The model under review builds one solid part; all positions refer to its coordinate system, in mm. A direction names the side the tool comes from. Give positions to 0.01 mm unless a question says otherwise; leave off trailing zeros. Loops run counter-clockwise (first coordinate to the right, second up) from the corner with the lowest first, then second, coordinate; pieces in that order, holes last. Notation, with made-up numbers: M 59.5,44.5 L 105.5,44.5 A31 ccw 105.5,72.5 Z; hole C 51,5 d2. An arc over 180 degrees is marked long. One line per item, written item: value. Start each with the question number.
Q1. To check wall thickness, follow line 1 along Y through (x, z) = (0, 5); line 2 along Z through (x, y) = (4.5, -14); line 3 along Y through (x, z) = (4.5, 2). State the ranges of each line that lie inside material, in increasing order. Write a range as from..to.
Q2. For pin 1 (1.6 mm diameter, centred on y = -1.21, z = 2.5, fed in from +X), flat-tipped, find the tip position at first contact; note if it passes through.
Q3. We need section A-A on x = 4.5. Write out the cut boundary in (y, z), plus the area to 3 significant figures.
Q4. We need section B-B on z = 7.5. Give the number of separate pieces and of enclosed holes in the cut face, plus the area to 3 significant figures.
Q5. Mouldability with a two-part tool opening along X and no side actions: class faces 1 (the face through (13.5, -3, 4)), 2 (the face through (-1, 0.32, 4.44)), 3 (the face through (4, 0, 0)) as released by +X, released by -X, zero draft, split by the parting line, or undercut.
Q6. For faces 4 (the face through (11, -1, 3)), 5 (the face through (13.199, 2.215, 4.437)), 6 (the face through (4.61, -13.21, 2.72)), list the 3-axis set-ups (+Z, -Z, +X, -X, +Y, -Y) from which the entire face can be reached by the end or side of a thin tool; tool diameter is ignored.
Autodesk Inventor part; units mm, degrees
ref_plane "Work Plane1" through (0, -22.25, 0) normal (0, 1, 0) x (1, 0, 0)
ref_plane "YZ Plane" through (0, 0, 0) normal (1, 0, 0) x (0, 1, 0)
ref_plane "XZ Plane" through (0, 0, 0) normal (0, 1, 0) x (-1, 0, 0)
sketch "Sketch1" plane through (0, 0, 0) normal (0, 0, 1) x (1, 0, 0)
  circle A0 centre (9, 0) radius 1
  circle A1 centre (0, 0) radius 1
  line L0 (0, 2.5) -> (9, 2.5)
  arc A2 (0, 2.5) -> (-2.5, 0) centre (0, 0) ccw
  arc A3 (11.5, 0) -> (9, 2.5) centre (9, 0) ccw
  arc A4 (-3.2143, -2.5754) -> (-2.5, 0) centre (-7.5, 0) ccw
  arc A5 (11.5, 0) -> (12.2143, -2.5754) centre (16.5, 0) ccw
  arc A6 (-3.2143, -2.5754) -> (-4.1458, -4.7111) centre (4.5, -7.2111) ccw
  line L1 (-8.5, -4.7111) -> (-4.1458, -4.7111)
  line L2 (13.1458, -4.7111) -> (17.5, -4.7111)
  line L3 (17.5, -9.7111) -> (13.1458, -9.7111)
  line L4 (-4.1458, -9.7111) -> (-8.5, -9.7111)
  line L5 (17.5, -7.9611) -> (10.4529, -7.9611)
  line L6 (-1.4529, -7.9611) -> (-8.5, -7.9611)
  line L7 (-8.5, -6.4611) -> (-1.4529, -6.4611)
  line L8 (10.4529, -6.4611) -> (17.5, -6.4611)
  arc A7 (-4.1458, -9.7111) -> (13.1458, -9.7111) centre (4.5, -7.2111) ccw
  arc A8 (13.1458, -4.7111) -> (12.2143, -2.5754) centre (4.5, -7.2111) ccw
  arc A9 (-1.4529, -7.9611) -> (10.4529, -7.9611) centre (4.5, -7.2111) ccw
  arc A10 (10.4529, -6.4611) -> (-1.4529, -6.4611) centre (4.5, -7.2111) ccw
  line L9 (17.5, -4.7111) -> (17.5, -6.4611)
  line L10 (17.5, -7.9611) -> (17.5, -9.7111)
  line L11 (-8.5, -9.7111) -> (-8.5, -7.9611)
  line L12 (-8.5, -6.4611) -> (-8.5, -4.7111)
extrude "Extrusion1" add sketch "Sketch1" along normal blind 5
sketch "Sketch2" plane through (13.1458, -9.7111, 0) normal (0, -1, 0) x (1, 0, 0)
  line L0 (4.3542, 0) -> (4.3542, 5)
  line L1 (0, 0) -> (0, 5)
  circle A0 centre (2.1771, 2.5) radius 0.9
  circle A1 centre (-19.4687, 2.5) radius 0.9
  point P0 (-13.1458, 0)
  dimension "d13" = 1.8
extrude "Extrusion2" cut sketch "Sketch2" against normal blind 5
fillet "Fillet1" radius 0.8 8 edges at (17.5, -4.7111, 2.5) (17.5, -9.7111, 2.5) (-8.5, -4.7111, 2.5) (-8.5, -9.7111, 2.5) (17.5, -6.4611, 2.5) (17.5, -7.9611, 2.5) (-8.5, -7.9611, 2.5) (-8.5, -6.4611, 2.5)
fillet "Fillet2" radius 0.8 4 edges at (-1.4529, -6.4611, 2.5) (10.4529, -6.4611, 2.5) (10.4529, -7.9611, 2.5) (-1.4529, -7.9611, 2.5)
sketch "Sketch3" plane through (0, 0, 5) normal (0, 0, 1) x (1, 0, 0)
  arc A0 (11.5, 0) -> (9, 2.5) centre (9, 0) ccw
  line L0 (14.4229, -6.4611) -> (14.4229, -4.7111)
  line L1 (9, 2.5) -> (14.4229, 2.5)
  line L2 (14.4229, 2.5) -> (14.4229, -4.7111)
  line L3 (14.4229, -4.7111) -> (9, -4.7111)
  line L4 (9, -4.7111) -> (9, 2.5)
  arc A1 (13.1458, -4.7111) -> (12.2143, -2.5754) centre (4.5, -7.2111) ccw
  arc A2 (11.5, 0) -> (12.2143, -2.5754) centre (16.5, 0) ccw
  point P0 (0, 0)
extrude "Extrusion3" add sketch "Sketch3" against normal blind 5 contours A0 L1 L2 L3 A1 A2
sketch "Sketch4" plane through (14.4229, -4.7111, 5) normal (1, 0, 0) x (0, 0, -1)
  line L0 (0, 0) -> (0, 7.2111)
  line L1 (2.5, 0) -> (0, 0)
  line L2 (5, 0) -> (2.5, 0)
  line L3 (5, 7.2111) -> (5, 0)
  line L4 (0, 7.2111) -> (5, 7.2111)
  point P0 (5, 4.7111)
extrude "Extrusion4" cut sketch "Sketch4" against normal blind 0.923
sketch "Sketch5" plane through (13.4999, -4.7111, 5) normal (1, 0, 0) x (0, 0, -1)
  line L0 (0, 3.5) -> (5, 3.5)
  circle A0 centre (2.5, 3.5) radius 0.9
  point P0 (5, 4.7111)
  dimension "d25" = 1.8
extrude "Extrusion5" cut sketch "Sketch5" against normal blind 2.5
fillet "Fillet3" radius 1 1 edges at (13.4999, 2.5, 2.5)
sketch "Sketch6" plane through (0, 0, 5) normal (0, 0, 1) x (1, 0, 0)
  arc A0 (-1.342, -8.5787) -> (10.342, -8.5787) centre (4.5, -7.2111) ccw
  circle A1 centre (4.5, -7.2111) radius 6
  circle A2 centre (4.5, -7.2111) radius 9
  line L0 (13.4999, -4.7111) -> (13.4999, 1.5)
  line L1 (13.4999, -4.7111) -> (17.88, -4.7111)
  line L2 (17.88, -4.7111) -> (17.88, -10.4948)
  line L3 (17.88, -10.4948) -> (13.4999, -10.4948)
  line L4 (13.4999, -10.4948) -> (13.4999, -4.7111)
  line L5 (-4.1458, -4.7111) -> (-7.7, -4.7111)
  line L6 (-4.1458, -4.7111) -> (-9.7441, -4.7111)
  line L7 (-9.7441, -4.7111) -> (-9.7441, -9.7121)
  line L8 (-9.7441, -9.7121) -> (-4.1458, -9.7121)
  line L9 (-4.1458, -9.7121) -> (-4.1458, -4.7111)
  line L10 (13.4999, -10.4948) -> (12.8796, -10.4948)
  point P0 (0, 0)
  point P1 (-4.1458, -9.7111)
  point P2 (13.4999, -7.1696)
extrude "Extrusion6" cut sketch "Sketch6" against normal blind 10 contours L4 L10 A2 | L4 L1 L2 L3 | A2 L8 L7 L6 L5
sketch "Sketch7" plane through (0, 0, 5) normal (0, 0, 1) x (1, 0, 0)
  arc A0 (-1.342, -8.5787) -> (10.342, -8.5787) centre (4.5, -7.2111) ccw
  circle A1 centre (4.5, -7.2111) radius 6
  circle A2 centre (4.5, -7.2111) radius 9
  line L0 (-4.4687, -6.4611) -> (-2.121, -6.4611)
  arc A3 (-2.121, -6.4611) -> (-1.342, -5.8435) centre (-2.121, -5.6611) ccw
  line L1 (-2.121, -7.9611) -> (-4.4687, -7.9611)
  arc A4 (-1.342, -8.5787) -> (-2.121, -7.9611) centre (-2.121, -8.7611) ccw
  line L2 (11.121, -6.4611) -> (13.4999, -6.4611)
  arc A5 (10.342, -5.8435) -> (11.121, -6.4611) centre (11.121, -5.6611) ccw
  arc A6 (11.121, -7.9611) -> (10.342, -8.5787) centre (11.121, -8.7611) ccw
  line L3 (13.4687, -7.9611) -> (11.121, -7.9611)
  point P0 (0, 0)
  point P1 (13.4687, -6.4611)
  point P2 (10.342, -8.5787)
  point P3 (-1.342, -8.5787)
extrude "Extrusion7" add sketch "Sketch7" against normal up to surface (5 mm away) contours A4 L1 A2 L0 A3 A1 | A1 A5 L2 A2 L3 A6
sketch "Sketch8" plane through (0, 0, 5) normal (0, 0, 1) x (1, 0, 0)
  circle A0 centre (4.5, -7.2111) radius 6
  circle A1 centre (0, 0) radius 1
  circle A2 centre (9, 0) radius 1
  arc A3 (-3.2143, -2.5754) -> (13.4687, -6.4611) centre (4.5, -7.2111) ccw
  line L0 (13.4687, -6.4611) -> (13.4999, -6.4611)
  line L1 (13.4999, -6.4611) -> (13.4999, 1.5)
  arc A4 (13.4999, 1.5) -> (12.4999, 2.5) centre (12.4999, 1.5) ccw
  line L2 (12.4999, 2.5) -> (0, 2.5)
  arc A5 (0, 2.5) -> (-2.5, 0) centre (0, 0) ccw
  arc A6 (-3.2143, -2.5754) -> (-2.5, 0) centre (-7.5, 0) ccw
extrude "Extrusion8" add sketch "Sketch8" along normal blind 4
ref_plane "Work Plane1" through (0, -22.25, 0) normal (0, 1, 0) x (1, 0, 0)
sketch "Sketch9" plane through (0, -22.25, 0) normal (0, 1, 0) x (1, 0, 0)
  line L0 (-4.5, -9) -> (13.5, -9)
  line L1 (13.5, 0) -> (13.5, -9)
  circle A0 centre (4.5, -4.5) radius 1.4
  point P0 (0, 0)
  point P1 (-3.2143, -9)
  point P2 (13.4687, -9)
  dimension "d36" = 2.8
extrude "Extrusion9" cut sketch "Sketch9" along normal blind 10
chamfer "Chamfer2" distance 0.5 angle 45 2 edges at (4.5, -13.2111, 0) (-1.5, -7.2111, 9)
sketch "Sketch10" plane through (0, 0, 0) normal (0, 0, -1) x (-1, 0, 0)
  circle A0 centre (0, 0) radius 1.05
  circle A1 centre (-9, 0) radius 1
  circle A2 centre (-9, 0) radius 1.05
  dimension "d42" = 2.1
  dimension "d43" = 2.1
extrude "Extrusion10" cut sketch "Sketch10" against normal blind 10
chamfer "Chamfer3" distance 0.5 angle 45 4 edges at (1.05, 0, 0) (10.05, 0, 0) (1.05, 0, 9) (10.05, 0, 9)
properties part number "hold pen - slider pen"
Solved:
1. line 1: -15.01..-11.18, -3.24..-1.05, 1.05..2.5
1. line 2: 0..3.1, 5.9..9
1. line 3: -16.21..-13.21, -1.21..2.5
2. pin 1: x = 11
3. outline: M -16.21,0 L -13.71,0 L -13.21,0.5 L -13.21,3.1 L -16.21,3.1 Z; M -16.21,5.9 L -13.21,5.9 L -13.21,8.5 L -13.71,9 L -16.21,9 Z; M -1.21,0.5 L -0.71,0 L 2.5,0 L 2.5,9 L -0.71,9 L -1.21,8.5 Z
3. area: 51.5 mm2
4. separate pieces: 1
4. enclosed holes: 3
4. area: 169 mm2
5. face 1: released by +X
5. face 2: undercut
5. face 3: zero draft
6. face 4: +X
6. face 5: +Z, -Z, +X, +Y
6. face 6: +Z, -Z
